Could you check a few things on this model? Use its own coordinates, in mm. Face numbers are marked on the shaded views. Round coordinates to 2 decimals unless told otherwise and drop trailing zeros. Loops run counter-clockwise (first coordinate to the right, second up) from the corner with the lowest first, then second, coordinate; pieces in that order, holes last. Notation, with made-up numbers: M 66,44 L 75,44 A19 cw 75,75 Z; hole C -26,2.25 d7. An arc over 180 degrees is marked long. One line per item, written item: value. Start each with the question number.
Q1. Please list where these lines run through material, in increasing order: line 1 along X through (y, z) = (-17.5, -18); line 2 along Y through (x, z) = (14.5, 0); line 3 along Y through (x, z) = (-1.25, 0).
Q2. Imagine slicing it at B-B (x = 5.25). Give the number of separate pieces and of enclosed holes in the cut face, then the cut area to 3 significant figures.
Q3. Thinking about a two-plate mould opening in Z: for the marked faces 1 and 2, which applies, released by +Z, released by -Z, zero draft, split by the parting line, or undercut?
Q4. I'm going to push flat-ended pins straight in: pin 1 Ø15.5 at (y, z) = (12.5, 0) entering from -X; pin 2 Ø8 at (x, y) = (12, -6) entering from -Z; pin 3 Ø1.5 at (x, z) = (-1, 14.5) entering from +Y. Where does each tip first touch, or does it pass through?
Q5. Imagine slicing it at A-A (x = -5). Please give me the cut outline in (y, z), then the cut area to 3 significant figures.
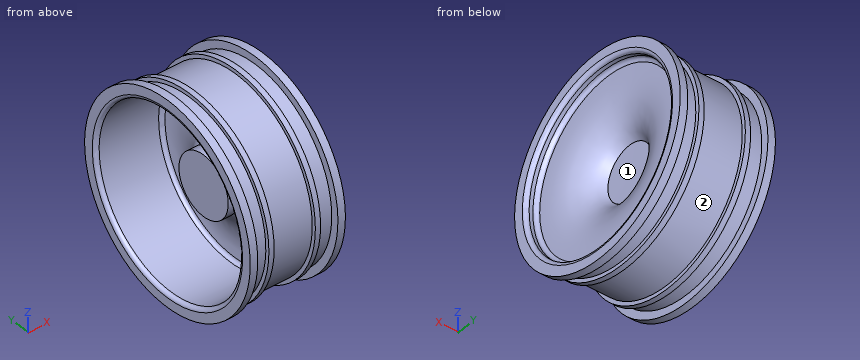
from build123d import *


with BuildPart() as f1:
    # F0 (on Front) → F1 (revolve)
    with BuildSketch(Plane.XZ):
        with BuildLine():
            Line((0, 8), (0, 0))
            Line((0, 0), (7.053804, 0))
            Line((7.053804, 0), (7.10286, 7.121615))
            add(Edge.make_bspline(
                [(12.751287, 22.386151), (12.729504, 17.395303), (12.390139, 10.323073), (7.10286, 7.121615)],
                knots=[1.104509, 1.104509, 1.104509, 1.104509, 17.208148, 17.208148, 17.208148, 17.208148], degree=3))
            ThreePointArc((12.751287, 22.386151), (13.045715, 23.090435), (13.751277, 23.381786))
            Line((13.751277, 23.381786), (14.752781, 23.381786))
            ThreePointArc((14.752781, 23.381786), (15.459887, 23.67468), (15.752781, 24.381786))
            Line((15.752781, 24.381786), (15.752781, 26.881786))
            Line((15.752781, 26.881786), (13.752781, 26.881786))
            Line((13.752781, 26.881786), (13.752781, 24.881786))
            Line((13.752781, 24.881786), (9.952781, 24.881786))
            Line((9.952781, 24.881786), (9.952781, 25.881786))
            Line((9.952781, 25.881786), (8.552781, 25.881786))
            Line((8.552781, 25.881786), (8.552781, 24.881786))
            Line((8.552781, 24.881786), (-2.447219, 24.881786))
            Line((-2.447219, 24.881786), (-2.447219, 25.881786))
            Line((-2.447219, 25.881786), (-3.847219, 25.881786))
            Line((-3.847219, 25.881786), (-3.847219, 24.881786))
            Line((-3.847219, 24.881786), (-7.647219, 24.881786))
            Line((-7.647219, 24.881786), (-7.647219, 26.881786))
            Line((-7.647219, 26.881786), (-9.647219, 26.881786))
            Line((-9.647219, 26.881786), (-9.647219, 24.381786))
            ThreePointArc((-9.647219, 24.381786), (-9.354326, 23.67468), (-8.647219, 23.381786))
            Line((-8.647219, 23.381786), (7.235566, 23.381786))
            ThreePointArc((7.235566, 23.381786), (7.88993, 23.137966), (8.2252, 22.525401))
            add(Edge.make_bspline(
                [(8.2252, 22.525401), (8.952293, 17.515068), (7.575597, 10.359274), (2.874941, 8)],
                knots=[0.897887, 0.897887, 0.897887, 0.897887, 16.237359, 16.237359, 16.237359, 16.237359], degree=3))
            Line((2.874941, 8), (0, 8))
        make_face()
    revolve(axis=Axis((3.526902, 0, 0), (-1, 0, 0)))


solid = f1.part
Report:
1. line 1: x = -9.65 to -7.65, -3.85 to -2.45, 8.55 to 9.95, 13.75 to 15.75
1. line 2: y = -26.88 to -23.38, 23.38 to 26.88
1. line 3: y = -24.88 to -23.38, 23.38 to 24.88
2. separate pieces: 2
2. enclosed holes: 1
2. area: 534 mm²
3. face 1: undercut
3. face 2: split by the parting line
4. pin 1: stops at x = 0
4. pin 2: stops at z = -26.77
4. pin 3: stops at y = 20.74
5. outline: C 0,0 d49.76; hole C 0,0 d46.76
5. area: 227 mm²
